Read the model definition and answer for the solid it produces. Units are mm, in the model's axes. A direction names the side the tool comes from. Give positions to 0.01 mm unless a question says otherwise; leave off trailing zeros. Loops run counter-clockwise (first coordinate to the right, second up) from the corner with the lowest first, then second, coordinate; pieces in that order, holes last. Notation, with made-up numbers: M -19.5,83 L -10.5,83 A9 ccw -10.5,90 Z; hole C -9,33.25 d2. An arc over 180 degrees is marked long. Return JSON: item names as keys, results as strings. Group by question number.
```python
from build123d import *

# Parameters (mm, degrees)
BOSS_EXTRUDE1_DEPTH     = 15
CUT_EXTRUDE4_START      = -3
SKETCH4_R               = 3
SKETCH4_R_2             = 1.75
CUT_EXTRUDE4_DEPTH      = 15
SKETCH4_2_R             = 1.75
CUT_EXTRUDE5_DEPTH      = 12.5000001
CUT_EXTRUDE5_DEPTH_BACK = 12.5000001
CUT_EXTRUDE6_START      = 3
CUT_EXTRUDE6_DEPTH      = 15
SKETCH6_R               = 14
CUT_EXTRUDE7_DEPTH      = 6.8
SKETCH7_W               = 12
SKETCH7_H               = 3
BOSS_EXTRUDE2_DEPTH     = 8
FILLET1_R               = 1
CHAMFER2_SIZE           = 0.2


with BuildPart() as part:
    # Sketch1 → Boss-Extrude1 (new body)
    with BuildSketch(Plane.XY):
        with BuildLine():
            Line((1.1, 11.447270417), (1.1, 4.156921938))
            ThreePointArc((1.1, 4.156921938), (3.407345007, 2.62297541), (4.3, 0))
            ThreePointArc((4.3, 0), (-2.62297541, -3.407345007), (-1.1, 4.156921938))
            Line((-1.1, 4.156921938), (-1.1, 11.447270417))
            ThreePointArc((-1.1, 11.447270417), (-7.733045972, -8.511756575), (11.5, 0))
            ThreePointArc((11.5, 0), (8.511756575, 7.733045972), (1.1, 11.447270417))
        make_face()
    extrude(amount=BOSS_EXTRUDE1_DEPTH)

    # Sketch4 → Cut-Extrude4 (cut)
    with BuildSketch(Plane(origin=(0, 0, 0), x_dir=(0, 0, -1), z_dir=(1, 0, 0)).offset(CUT_EXTRUDE4_START)):
        with Locations((-11.5, 7)):
            Circle(SKETCH4_R)
        with Locations((-11.5, 7)):
            Circle(SKETCH4_R_2, mode=Mode.SUBTRACT)
        with Locations((-3.5, 7)):
            Circle(SKETCH4_R)
        with Locations((-3.5, 7)):
            Circle(SKETCH4_R_2, mode=Mode.SUBTRACT)
    extrude(amount=-CUT_EXTRUDE4_DEPTH, mode=Mode.SUBTRACT)

    # Sketch4_2 → Cut-Extrude5 (cut, two sides)
    with BuildSketch(Plane(origin=(0, 0, 0), x_dir=(0, 0, -1), z_dir=(1, 0, 0))) as cut_extrude5_sk:
        with Locations((-11.5, 7)):
            Circle(SKETCH4_2_R)
        with Locations((-3.5, 7)):
            Circle(SKETCH4_2_R)
    extrude(amount=CUT_EXTRUDE5_DEPTH, mode=Mode.SUBTRACT)
    extrude(cut_extrude5_sk.sketch, amount=-CUT_EXTRUDE5_DEPTH_BACK, mode=Mode.SUBTRACT)

    # Sketch5 → Cut-Extrude6 (cut)
    with BuildSketch(Plane(origin=(0, 0, 0), x_dir=(0, 0, -1), z_dir=(1, 0, 0)).offset(CUT_EXTRUDE6_START)):
        Polygon((-9.883419246, 9.8), (-13.116580754, 9.8), (-14.733161507, 7), (-13.116580754, 4.2), (-9.883419246, 4.2), (-8.266838493, 7), align=None)
        Polygon((-1.883419246, 9.8), (-5.116580754, 9.8), (-6.733161507, 7), (-5.116580754, 4.2), (-1.883419246, 4.2), (-0.266838493, 7), align=None)
    extrude(amount=CUT_EXTRUDE6_DEPTH, mode=Mode.SUBTRACT)

    # Sketch6 → Cut-Extrude7 (cut)
    with BuildSketch(Plane(origin=(0, 0, 0), x_dir=(-1, 0, 0), z_dir=(0, 0, -1))):
        Circle(SKETCH6_R)
    extrude(amount=-CUT_EXTRUDE7_DEPTH, mode=Mode.SUBTRACT)

    # Sketch7 → Boss-Extrude2 (add)
    with BuildSketch(Plane.XY.offset(15)):
        with Locations((17.401754251, 0)):
            Rectangle(SKETCH7_W, SKETCH7_H)
    extrude(amount=-BOSS_EXTRUDE2_DEPTH)

    # Fillet1
    fillet1_edges = [part.edges().sort_by_distance(p)[0] for p in [
        (11.401754251, -1.5, 11),
        (11.401754251, 1.5, 11),
        (23.401754251, 1.5, 11),
        (23.401754251, -1.5, 11),
    ]]
    fillet(fillet1_edges, radius=FILLET1_R)

    # Chamfer2
    chamfer2_edges = [part.edges().sort_by_distance(p)[0] for p in [
        (-8.549394828, -7.691413919, 15),
        (23.401754251, 0, 15),
        (17.324601482, -1.5, 15),
        (17.324601482, 1.5, 15),
        (7.691413919, 8.549394828, 15),
        (23.108861032, -1.207106781, 15),
        (23.108861032, 1.207106781, 15),
        (11.614993182, -1.725403331, 15),
        (11.614993182, 1.725403331, 15),
        (1.1, 7.802096178, 15),
        (0, -4.3, 15),
        (-1.1, 7.802096178, 15),
    ]]
    chamfer(chamfer2_edges, length=CHAMFER2_SIZE)


solid = part.part
```
1. Find section C-C (z = 7.5). Write down the section's boundary in (x, y), and give its area (3 significant figures).
2. Find section A-A (x = 17.5). Write down the section's boundary in (y, z), and give its area (3 significant figures).
3. Find section B-B (z = 11.5). Write down the section's boundary in (x, y).
4. For faces 1 (the flat face through (17, 1.5, 11)), 2 (the flat face through (7, 4.2, 12)), 3 (the cylindrical face through (-5.97, 4.07, 12.15)), determine the directions among +Z, -Z, +X, -X, +Y, -Y from which every point of the face is accessible in a straight line to the end or side of a thin tool.
5. Straight lines are drawn through the part: line 1 along X through (y, z) = (0, 10.25); line 2 along Z through (x, y) = (2.1, 7); line 3 along Y through (x, z) = (-2.1, 11.5). For each, find the intervals that lie inside material, in ascending order.
6. The mould has two halves that part along Z. Classify faces 4 (the flat face through (-3, 7, 9.5)), 5 (the flat face through (17, -1.5, 11)), 6 (the flat face through (17, 0, 7)): +Z half, -Z half, draft (parallel to the pull), parting line (faces both ways), or undercut.
7. Flat-ended cylindrical pins translate along their axes: P1, Ø3, axis at y = 8, z = 12, coming from the -X side; P2, Ø2, axis at x = 12, y = 5.5, coming from the -Z side; P3, Ø4.5, axis at y = 7, z = 11.5, coming from the +X side; P4, Ø5, axis at x = 14.5, y = 0.5, coming from the -Z side. Find the tip coordinate at first contact, or state that the pin passes through.
8. Find section D-D (x = 0). Write down the section's boundary in (y, z).
Result:
{
 "1": {"outline": "M -1.1,4.16 L -1.1,11.45 A11.5 ccw long 11.27,-2.3 A1 cw 12.25,-1.5 L 22.4,-1.5 A1 ccw 23.4,-0.5 L 23.4,0.5 A1 ccw 22.4,1.5 L 12.25,1.5 A1 cw 11.27,2.3 A11.5 ccw 1.1,11.45 L 1.1,4.16 A4.3 cw long Z", "area": "377 mm2"},
 "2": {"outline": "M -1.5,7 L 1.5,7 L 1.5,14.8 L 1.3,15 L -1.3,15 L -1.5,14.8 Z", "area": "24.0 mm2"},
 "3": {"outline": "M -10.78,4 A11.5 ccw long 11.27,-2.3 A1 cw 12.25,-1.5 L 22.4,-1.5 A1 ccw 23.4,-0.5 L 23.4,0.5 A1 ccw 22.4,1.5 L 12.25,1.5 A1 cw 11.27,2.3 A11.5 ccw 10.71,4.2 L 3,4.2 L 3,5.25 L 1.1,5.25 L 1.1,4.16 A4.3 cw long -1.1,4.16 L -1.1,5.25 L -3,5.25 L -3,4 Z; M -5.68,10 L -3,10 L -3,8.75 L -1.1,8.75 L -1.1,11.45 A11.5 ccw Z; M 1.1,8.75 L 3,8.75 L 3,9.8 L 6.02,9.8 A11.5 ccw 1.1,11.45 Z"},
 "4": {"face 1": "+Z, -Z, +X, +Y", "face 2": "+X", "face 3": "-X"},
 "5": {"line 1": "x = -11.5 to -4.3, 4.3 to 23.4", "line 2": "z = 6.8 to 9.75, 13.25 to 15", "line 3": "y = -11.31 to -3.75, 3.75 to 5.25, 8.75 to 11.31"},
 "6": {"face 4": "undercut", "face 5": "draft", "face 6": "-Z half"},
 "7": {"P1": "stops at x = -3", "P2": "passes through", "P3": "stops at x = 3", "P4": "stops at z = 7"},
 "8": {"outline": "M -11.5,6.8 L -4.3,6.8 L -4.3,14.8 L -4.5,15 L -11.3,15 L -11.5,14.8 Z"}
}
